Geometry check sheet. Reference: the model listing, model coordinates, mm. A direction names the side the tool comes from. Round coordinates to 2 decimals unless told otherwise and drop trailing zeros. Loops run counter-clockwise (first coordinate to the right, second up) from the corner with the lowest first, then second, coordinate; pieces in that order, holes last.
Autodesk Inventor part; units mm, degrees
ref_plane "YZ Plane" through (0, 0, 0) normal (1, 0, 0) x (0, 1, 0)
ref_plane "XZ Plane" through (0, 0, 0) normal (0, 1, 0) x (-1, 0, 0)
ref_plane "XY Plane" through (0, 0, 0) normal (0, 0, 1) x (1, 0, 0)
sketch "Sketch1" plane through (0, 0, 0) normal (0, 0, 1) x (1, 0, 0)
  line L0 (-1.633, 4.75) -> (-10.633, 4.75)
  line L1 (-10.633, 4.75) -> (-10.633, 11)
  line L2 (-10.633, 11) -> (-17.633, 11)
  line L3 (-17.633, 11) -> (-17.633, 0)
  line L4 (-17.633, 0) -> (8.367, 0)
  line L5 (-1.633, 4.75) -> (-1.633, 3)
  line L6 (-1.633, 3) -> (8.367, 3)
  line L7 (8.367, 3) -> (8.367, 0)
  point P0 (0, 0)
  dimension "d3" = 9
  dimension "d5" = 11
  dimension "d6" = 7
  dimension "d7" = 1.75
  dimension "d8" = 3
  dimension "d9" = 4.75
revolve "Revolution1" add sketch "Sketch1" angle 360 about axis through (-17.633, 0, 0) along (1, 0, 0)
properties part number "guia"
1) Gauge pin test, flat ends, axial feed: pin 1 (5 mm diameter, centred on x = 0, y = 5.5, fed in from +Z); pin 2 (1.5 mm diameter, centred on y = -1, z = -7, fed in from +X); pin 3 (4 mm diameter, centred on x = -7, y = -0.5, fed in from -Z). Record the tip position at first contact, or that the pin passes through.
Report:
pin 1: stops at z = 3.09
pin 2: stops at x = -10.63
pin 3: stops at z = -4.75
2) Sectioned sample at A-A, the plane z = 0. Record the cut outline in (x, y), then the cut area to 4 significant figures.
Report:
outline: (-17.63, -11) - (-10.63, -11) - (-10.63, -4.75) - (-1.63, -4.75) - (-1.63, -3) - (8.37, -3) - (8.37, 3) - (-1.63, 3) - (-1.63, 4.75) - (-10.63, 4.75) - (-10.63, 11) - (-17.63, 11) - close
area: 299.5 mm2
3) Scan lines: line 1 along X through (y, z) = (-8, 4.25); line 2 along X through (y, z) = (2.75, -2); line 3 along Z through (x, y) = (-8.5, -4). Record each from-to range of solid material in increasing order.
Report:
line 1: x = -17.63 to -10.63
line 2: x = -17.63 to -1.63
line 3: z = -2.56 to 2.56
4) Access from +Z, -Z, +X, -X, +Y, -Y to the whole of each face (thin tool, end or side, straight path). Record for faces 1 (the face through (-6.196, 2.192, 4.214)), 2 (the face through (-14.18, -2.38, 10.74)).
Report:
face 1: +X
face 2: +X, -X
5) Sectioned sample at D-D, the plane x = -14. Record the cut outline in (y, z), then the cut area to 3 significant figures.
Report:
outline: circle Ø22 at (0, 0)
area: 380 mm2
6) Sectioned sample at C-C, the plane x = 4. Record the cut outline in (y, z).
Report:
outline: circle Ø6 at (0, 0)
